Input: part model. Units: mm. Frame: model coordinates. Coordinates: 2 decimals unless noted, no trailing zeros. Order: outer loops, then holes, each group sorted by start corner. A loop starts at its lowest first (then second) coordinate and runs counter-clockwise, first axis right, second up.
from build123d import *

# Parameters (mm, degrees)
SM_BASE_FLANGE_2_DEPTH = 30
HOLE_WIZARD_M3_1_D     = 3.2
SKETCH_24_R            = 6.1
CUT_EXTRUDE_2_DEPTH    = 103.08329932
HOLE_WIZARD_M4_1_D     = 4.3
HOLE_WIZARD_M2_1_D     = 2.2
HOLE_WIZARD_M3_1_2_D   = 3.15


# Sheet-metal steps are written as plain solids
with BuildPart() as part:
    # 草圖16 → 基材-凸緣2 (new, symmetric)
    with BuildSketch(Plane.XY):
        with BuildLine():
            Line((40, 0), (0.7366, 0))
            ThreePointArc((0.7366, 0), (0.215745145, 0.215745145), (0, 0.7366))
            Line((0, 0.7366), (0, 85))
            Line((0, 85), (-4, 85))
            Line((-4, 85), (-4, 0.7366))
            ThreePointArc((-4, 0.7366), (-2.61268198, -2.61268198), (0.7366, -4))
            Line((0.7366, -4), (40, -4))
            Line((40, -4), (40, 0))
        make_face()
    extrude(amount=SM_BASE_FLANGE_2_DEPTH, both=True)

    # Hole Wizard M3 _1 (through all)
    with Locations(Plane(origin=(0, 0, 0), x_dir=(-1, 0, 0), z_dir=(0, 1, 0))):
        with Locations((-27, 27.5), (-11, 12.5), (-11, 27.5), (-27, 12.5)):
            Hole(HOLE_WIZARD_M3_1_D / 2)

    # 草圖24 → 除料-伸長2 (cut, through all)
    with BuildSketch(Plane.XZ.offset(4)):
        with Locations(Location((19, 0, 0), (0, 0, 270))):
            Circle(SKETCH_24_R)
    extrude(amount=-CUT_EXTRUDE_2_DEPTH, mode=Mode.SUBTRACT)

    # M4 餘隙孔1 (through all)
    with Locations(Plane(origin=(0, 0, 0), x_dir=(0, 0, 1), z_dir=(1, 0, 0))):
        with Locations((10, -81), (25, -81), (25, -61), (10, -61)):
            Hole(HOLE_WIZARD_M4_1_D / 2)

    # M2 餘隙孔1 (through all)
    with Locations(Plane(origin=(0, -4, 0), x_dir=(-1, 0, 0), z_dir=(0, -1, 0))):
        with Locations((-14, 0), (-24, 0)):
            Hole(HOLE_WIZARD_M2_1_D / 2)

    # Hole Wizard M3 _1 2 (through all)
    with Locations(Plane(origin=(0, -4, 0), x_dir=(-1, 0, 0), z_dir=(0, -1, 0))):
        with Locations((-26.75, -6.423393759), (-34.5, 7), (-3.5, 7), (-11.25, -6.423393759), (-11.25, 20.423393759), (-26.75, 20.423393759)):
            Hole(HOLE_WIZARD_M3_1_2_D / 2)


solid = part.part
Item 1: Draft query along Y for faces 1 (the face through (-2.03, 63.1, 10.47)), 2 (the face through (-2, 85, 0)), 3 (the face through (0, 42, 0)), 4 (the face through (-2.03, 82.91, 24.01)). Return one class per face: pulls with the +Y half, pulls with the -Y half, needs draft (parallel to the pull), parting line crosses it, or undercut.
Response values:
face 1: undercut
face 2: pulls with the +Y half
face 3: needs draft
face 4: undercut
Item 2: Cut plane A-A on x = 19. Return loops of the section in (y, z), then the cut area to 3 significant figures.
Response values:
outline: (-4, -30) - (0, -30) - (0, -6.1) - (-4, -6.1) - close; (-4, 6.1) - (0, 6.1) - (0, 30) - (-4, 30) - close
area: 191 mm2
Item 3: Cut plane D-D on z = 19. Return loops of the section in (x, y).
Response values:
outline: (-4, 0.74) arc R4.74 ccw to (0.74, -4) - (40, -4) - (40, 0) - (0.74, 0) arc R0.74 cw to (0, 0.74) - (0, 85) - (-4, 85) - close
Item 4: Ray query, probe 1 along Z at (x, y) = (27, -3); probe 2 along Z at (x, y) = (-1, 61); probe 3 along Z at (x, y) = (26.75, -0.8). Return the intervals inside material, ascending.
Response values:
probe 1: z = -30 to -21.98, -18.87 to 4.87, 7.98 to 10.9, 14.1 to 25.9, 29.1 to 30
probe 2: z = -30 to 7.85, 12.15 to 22.85, 27.15 to 30
probe 3: z = -30 to -22, -18.85 to 4.85, 8 to 10.92, 14.08 to 25.92, 29.08 to 30
Item 5: Pin query (flat end, axial travel): pin 1 Ø7 at (y, z) = (81, 10) entering from +X; pin 2 Ø5 at (x, z) = (10.5, -0.5) entering from +Y; pin 3 Ø4 at (x, z) = (27, 27.5) entering from -Y. Return the tip coordinate at first contact, or that it passes through.
Response values:
pin 1: stops at x = 0
pin 2: stops at y = 0
pin 3: stops at y = -4
Item 6: Cut plane B-B on z = 0. Return loops of the section in (x, y), then the cut area to 3 significant figures.
Response values:
outline: (-4, 0.74) arc R4.74 ccw to (0.74, -4) - (12.9, -4) - (12.9, 0) - (0.74, 0) arc R0.74 cw to (0, 0.74) - (0, 85) - (-4, 85) - close; (25.1, -4) - (40, -4) - (40, 0) - (25.1, 0) - close
area: 463 mm2
Item 7: Cut plane C-C on y = 61. Return loops of the section in (x, z), then the cut area to 3 significant figures.
Response values:
outline: (-4, -30) - (0, -30) - (0, 7.85) - (-4, 7.85) - close; (-4, 12.15) - (0, 12.15) - (0, 22.85) - (-4, 22.85) - close; (-4, 27.15) - (0, 27.15) - (0, 30) - (-4, 30) - close
area: 206 mm2
